from build123d import *

# Parameters (mm, degrees)
SKETCH_1_R      = 45
SKETCH_1_R_2    = 1.75
EXTRUDE_1_DEPTH = 2.6
SKETCH_3_R      = 34
SKETCH_2_R      = 35.5
SKETCH_4_R      = 34
EXTRUDE_2_DEPTH = 32.4
FILLET_1_R      = 10
EXTRUDE_3_DEPTH = 10
EXTRUDE_4_DEPTH = 20
SKETCH_7_R      = 36
SKETCH_7_R_2    = 27.5
EXTRUDE_5_DEPTH = 3
FILLET_2_R      = 10


with BuildPart() as part:
    # 草图1 → 凸台-拉伸1 (new body)
    with BuildSketch(Plane(origin=(0, 0, 0), x_dir=(1, 0, 0), z_dir=(0, 1, 0))):
        with Locations(Location((0, 0, 0), (0, 0, 270))):
            Circle(SKETCH_1_R)
        with Locations(Location((41.5, 0, 0), (0, 0, 270))):
            Circle(SKETCH_1_R_2, mode=Mode.SUBTRACT)
        with Locations(Location((-41.5, 0, 0), (0, 0, 270))):
            Circle(SKETCH_1_R_2, mode=Mode.SUBTRACT)
        with Locations(Location((0, 41.5, 0), (0, 0, 270))):
            Circle(SKETCH_1_R_2, mode=Mode.SUBTRACT)
        with Locations(Location((0, -41.5, 0), (0, 0, 270))):
            Circle(SKETCH_1_R_2, mode=Mode.SUBTRACT)
    extrude(amount=EXTRUDE_1_DEPTH)

    # 草图3 → 放样1 section 0
    with BuildSketch(Plane(origin=(0, -18, 0), x_dir=(-1, 0, 0), z_dir=(0, -1, 0))):
        Circle(SKETCH_3_R)
    # 草图2 → 放样1 section 1
    with BuildSketch(Plane.XZ):
        Circle(SKETCH_2_R)
    loft()

    # 草图4 → 凸台-拉伸2 (add)
    with BuildSketch(Plane.XZ.offset(18)):
        with Locations(Location((0, 0, 0), (0, 0, 270))):
            Circle(SKETCH_4_R)
    extrude(amount=EXTRUDE_2_DEPTH)

    # 圆角1
    fillet_1_edges = [part.edges().sort_by_distance(p)[0] for p in [
        (0, -50.4, 34),
    ]]
    fillet(fillet_1_edges, radius=FILLET_1_R)

    # 草图5 → 凸台-拉伸3 (add)
    with BuildSketch(Plane.XZ):
        Polygon((-17.67766953, 33.234018716), (-33.234018716, 17.67766953), (-37.476659403, 21.920310217), (-21.920310217, 37.476659403), align=None)
    extrude(amount=EXTRUDE_3_DEPTH)

    # 草图6 → 凸台-拉伸4 (add)
    with BuildSketch(Plane(origin=(-29.69848481, 0, 29.69848481), x_dir=(0.7071067811865436, 0, 0.7071067811865515), z_dir=(-0.7071067811865515, 0, 0.7071067811865436))):
        with BuildLine():
            Line((-7.5, -2), (7.5, -2))
            ThreePointArc((7.5, -2), (10.5, -5), (7.5, -8))
            Line((7.5, -8), (-7.5, -8))
            ThreePointArc((-7.5, -8), (-10.5, -5), (-7.5, -2))
        make_face()
    extrude(amount=EXTRUDE_4_DEPTH)

    # 草图7 → 凸台-拉伸5 (add)
    with BuildSketch(Plane(origin=(0, 2.6, 0), x_dir=(1, 0, 0), z_dir=(0, 1, 0))):
        with Locations(Location((0, 0, 0), (0, 0, 270))):
            Circle(SKETCH_7_R)
        with Locations(Location((0, 0, 0), (0, 0, 270))):
            Circle(SKETCH_7_R_2, mode=Mode.SUBTRACT)
    extrude(amount=EXTRUDE_5_DEPTH)

    # 圆角2
    # the kernel refuses this fillet: 10 mm, written as the material it takes off along each edge
    with BuildSketch(Plane(origin=(0, 5.6, 0), x_dir=(0, 0, 1), z_dir=(-1, 0, 0))) as fillet_2_piece_1:
        with BuildLine():
            CenterArc((28.858571571, -10), FILLET_2_R, 44.427004001, 45.572995999)
            Line((28.858571571, 0), (28.858571571, 0.2))
            Line((28.858571571, 0.2), (36, 0.2))
            Line((36, 0.2), (36.2, 0))
            ThreePointArc((36.2, 0), (36.2, -1.5), (36.142828569, -2.86))
            Line((36.142828569, -2.86), (36, -3))
        make_face()
    revolve(axis=Axis((0, 5.6, 0), (0, 1, 0)), mode=Mode.SUBTRACT)


solid = part.part
The model under review builds one solid part; all positions refer to its coordinate system, in mm. A direction names the side the tool comes from. Give positions to 0.01 mm unless a question says otherwise; leave off trailing zeros. Write each loop counter-clockwise with the first axis right and the second up, starting at its lowest first coordinate (ties: lowest second). Pieces come first, ordered by that corner, then holes.
1. Draft analysis for pull direction X (two halves, no side actions). For faces 6 (the cylindrical face through (-0.67, 1.282, -39.883)), 7 (the cylindrical face through (-17.235, 1.282, 41.569)), 8 (the flat face through (0, -50.4, 0)), state which applies: +X half, -X half, draft (parallel to the pull), parting line (faces both ways), or undercut.
2. Add section D-D, the plane y = -21.5. Write out the cut boundary in (x, z).
3. Tool access review of faces 1 (the flat face through (-35.326, -4.93, 19.769)), 2 (the cylindrical face through (39.79, 1.28, -0.38)), 3 (the cylindrical face through (33.71, -29.04, 4.43)), 4 (the flat face through (0, 2.6, 0)), 5 (the flat face through (-19.829, -4.93, 35.385)): name each direction out of +Z, -Z, +X, -X, +Y, -Y from which nothing blocks a thin tool from reaching the whole face with its end or side.
4. Add section A-A, the plane x = 0. Write out the cut boundary in (y, z), plus the area to 3 significant figures.
5. For P1, Ø12, axis at x = 17.5, z = 39.5, coming from the -Y side; P2, Ø16.5, axis at x = 0.5, z = -12, coming from the +Y side; P3, Ø8, axis at y = -42.5, z = -20, coming from the +X side, all flat-tipped, find the tip position at first contact; note any pin that passes through.
6. Add section C-C, the plane y = -3.5. Write out the cut boundary in (x, z).
7. Wall thickness on L1, parallel to X at y = 1, z = 0; L2, parallel to Y at x = -5, z = 38; L3, parallel to Z at x = -19, y = -3.5: over which ranges is each line inside the solid? List them lowest first.
8. Add section B-B, the plane z = -41.5. Write out the cut boundary in (x, y).
Worked answers:
1. face 6: undercut
1. face 7: parting line
1. face 8: draft
2. outline: circle Ø68 at (0, 0)
3. face 1: -X, -Y
3. face 2: +Y, -Y
3. face 3: -Y
3. face 4: +Y
3. face 5: +Z, -Y
4. outline: (-50.4, -24) arc R10 ccw to (-40.4, -34) - (-18, -34) - (0, -35.5) - (0, -39.75) - (2.6, -39.75) - (2.6, -36) arc R10 ccw to (5.6, -28.86) - (5.6, -27.5) - (2.6, -27.5) - (2.6, 27.5) - (5.6, 27.5) - (5.6, 28.86) arc R10 ccw to (2.6, 36) - (2.6, 39.75) - (0, 39.75) - (0, 35.5) - (-18, 34) - (-40.4, 34) arc R10 ccw to (-50.4, 24) - close; (0, -45) - (2.6, -45) - (2.6, -43.25) - (0, -43.25) - close; (0, 43.25) - (2.6, 43.25) - (2.6, 45) - (0, 45) - close
4. area: 3,660 mm2
5. P1: stops at y = 0
5. P2: stops at y = 2.6
5. P3: stops at x = 29.86
6. outline: (-50.98, 36.7) - (-36.84, 22.56) - (-37.48, 21.92) - (-33.23, 17.68) - (-17.68, 33.23) - (-21.92, 37.48) - (-22.56, 36.84) - (-36.7, 50.98) - close; circle Ø70.42 at (0, 0)
7. L1: x = -45 to -43.25, -39.75 to 39.75, 43.25 to 45
7. L2: y = 0 to 2.6
7. L3: z = -29.64 to 29.64, 31.91 to 34.56
8. outline: (-17.4, 0) - (-1.75, 0) - (-1.75, 2.6) - (-17.4, 2.6) - close; (1.75, 0) - (17.4, 0) - (17.4, 2.6) - (1.75, 2.6) - close
